Design review of the part shown in the three views and the two pictorial views. Dimensions are in mm from the part's minimum x, y and z. A direction names the side the tool comes from. Give positions to 0.01 mm unless a question says otherwise; leave off trailing zeros. Loops run counter-clockwise (first coordinate to the right, second up) from the corner with the lowest first, then second, coordinate; pieces in that order, holes last. Notation, with made-up numbers: M -3.5,-36 L 33.5,-36 A12 cw 33.5,-32 Z; hole C 21.25,-12 d5. An arc over 180 degrees is marked long. Return JSON: item names as keys, results as strings. Group by question number.
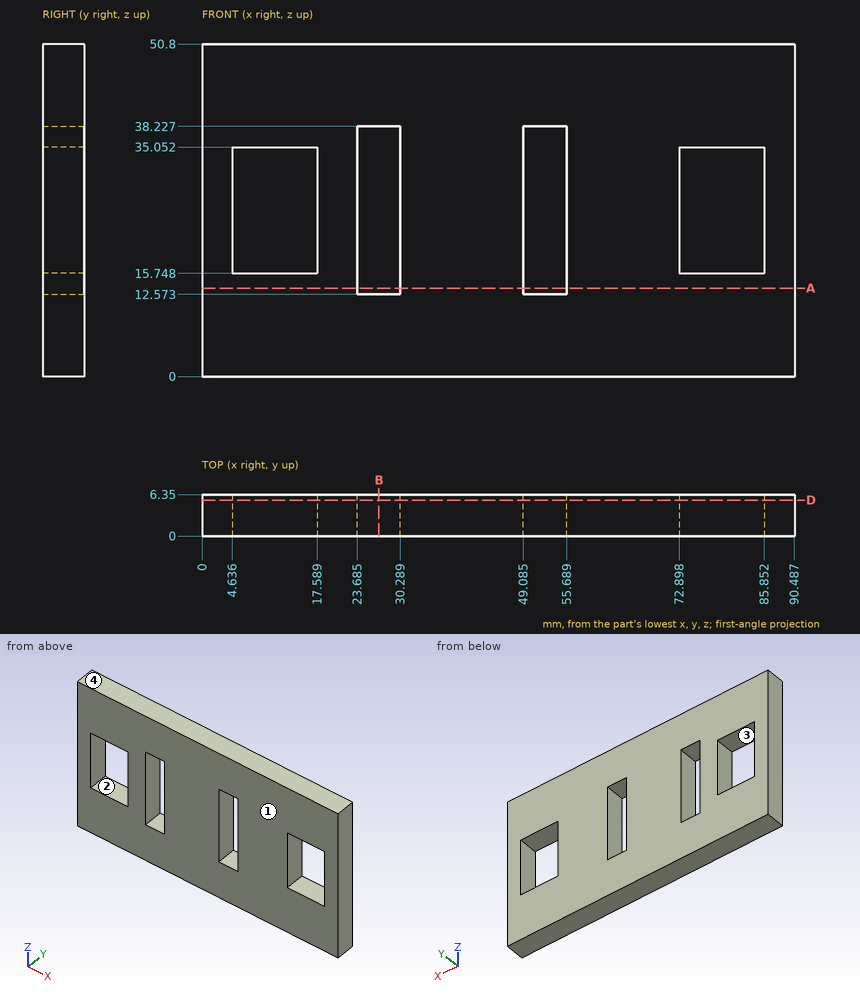
(1) Add section B-B (x = 27). Write out the cut boundary in (y, z).
(2) For the marked faces 1 and 2, list the 3-axis set-ups (+Z, -Z, +X, -X, +Y, -Y) from which the entire face can be reached by the end or side of a thin tool; tool diameter is ignored.
(3) Add section A-A (z = 13.5). Count the separate pieces of the cut face and the enclosed holes in it, and give its area (3 significant figures).
(4) For probe 1 along X at (y, z) = (6, 26.5) (1 decimal); probe 2 along X at (y, z) = (5.5, 36) (1 decimal); probe 3 along Z at (x, y) = (12.5, 5.5), list the stretches that pass through material, from the lowest coordinate up.
(5) Mouldability with a two-part tool opening along X and no side actions: class the marked faces 3 and 4 as released by +X, released by -X, zero draft, split by the parting line, or undercut.
(6) Add section D-D (y = 5.5). Write out the cut boundary in (x, z) (1 decimal), and give its area (3 significant figures).
Verdict:
{
 "1": {"outline": "M 0,0 L 6.35,0 L 6.35,12.57 L 0,12.57 Z; M 0,38.23 L 6.35,38.23 L 6.35,50.8 L 0,50.8 Z"},
 "2": {"face 1": "+Z, -Z, +X, -X, -Y", "face 2": "+Y, -Y"},
 "3": {"separate pieces": "3", "enclosed holes": "0", "area": "491 mm²"},
 "4": {"probe 1": "x = 0 to 4.6, 17.6 to 23.7, 30.3 to 49.1, 55.7 to 72.9, 85.9 to 90.5", "probe 2": "x = 0 to 23.7, 30.3 to 49.1, 55.7 to 90.5", "probe 3": "z = 0 to 15.75, 35.05 to 50.8"},
 "5": {"face 3": "undercut", "face 4": "zero draft"},
 "6": {"outline": "M 0,0 L 90.5,0 L 90.5,50.8 L 0,50.8 Z; hole M 4.6,15.7 L 17.6,15.7 L 17.6,35.1 L 4.6,35.1 Z; hole M 23.7,12.6 L 30.3,12.6 L 30.3,38.2 L 23.7,38.2 Z; hole M 49.1,12.6 L 55.7,12.6 L 55.7,38.2 L 49.1,38.2 Z; hole M 72.9,15.7 L 85.9,15.7 L 85.9,35.1 L 72.9,35.1 Z", "area": "3,760 mm²"}
}
